The listing builds one solid part. Answer for the finished solid, in the listing's coordinates (mm). Face numbers are marked on the shaded views. A direction names the side the tool comes from. Give positions to 0.01 mm unless a question says otherwise; leave off trailing zeros. Order: outer loops, then holes, each group sorted by start corner. A loop starts at its lowest first (then second) coordinate and runs counter-clockwise, first axis right, second up.
Autodesk Inventor part; units mm, degrees
ref_plane "YZ Plane" through (0, 0, 0) normal (1, 0, 0) x (0, 1, 0)
ref_plane "XZ Plane" through (0, 0, 0) normal (0, 1, 0) x (-1, 0, 0)
ref_plane "XY Plane" through (0, 0, 0) normal (0, 0, 1) x (1, 0, 0)
sketch "Sketch1" plane through (0, 0, 0) normal (0, 1, 0) x (-1, 0, 0)
  line L0 (0, 0) -> (41.148, 0)
  line L1 (41.148, 0) -> (41.148, -20.32)
  line L2 (41.148, -20.32) -> (0, -20.32)
  line L3 (0, -20.32) -> (0, 0)
  circle A0 centre (45.212, -15.24) radius 2.0193
  circle A1 centre (-4.064, -15.24) radius 2.0193
  circle A2 centre (45.212, -5.08) radius 2.0193
  circle A3 centre (-4.064, -5.08) radius 2.0193
  line L4 (41.148, -9.652) -> (49.276, -9.652)
  line L5 (41.148, -10.668) -> (49.276, -10.668)
  line L6 (-13.1318, -9.652) -> (0, -9.652)
  line L7 (-13.1318, -10.668) -> (0, -10.668)
  line L8 (-13.1318, 3.81) -> (49.276, 3.81)
  line L9 (49.276, 3.81) -> (49.276, -24.13)
  line L10 (49.276, -24.13) -> (-13.1318, -24.13)
  line L11 (-13.1318, -30.9945) -> (-13.1318, 13.2145)
  line L12 (-6.155, -5.4575) -> (-6.0508, -5.4409)
  line L13 (-6.155, -5.4575) -> (-6.0508, -5.4409)
  line L14 (20.574, -20.32) -> (20.574, 0)
  circle A4 centre (10.668, -10.16) radius 6.604
  circle A5 centre (-6.7818, 6.8645) radius 2.0193
  circle A6 centre (30.6451, 9.4045) radius 2.0193
  circle A7 centre (30.6451, -27.1845) radius 2.0193
  line L15 (10.668, -30.9945) -> (34.4551, -30.9945)
  line L16 (-8.128, -30.9945) -> (34.4551, -30.9945)
  circle A8 centre (-9.3218, -27.1845) radius 2.0193
  line L17 (34.4424, -30.9945) -> (-13.1318, -30.9945)
  line L18 (34.4424, -24.13) -> (34.4424, -30.9945)
  line L19 (34.4424, 13.2145) -> (34.4424, 3.81)
  circle A9 centre (30.6451, 9.4045) radius 2.286
  circle A10 centre (-6.7818, 6.8645) radius 2.286
  circle A11 centre (-9.3218, -27.1845) radius 2.286
  circle A12 centre (30.6451, -27.1845) radius 2.286
  line L20 (34.4424, 3.81) -> (-13.1318, 3.81)
  line L21 (34.4424, 13.2145) -> (-13.1318, 13.2145)
  point P0 (20.574, -10.16)
  point P1 (34.4424, -30.9945)
  point P2 (-11.5492, -24.13)
  point P3 (-7.0944, -24.13)
  dimension "d0" = 41.148
  dimension "d1" = 20.32
  dimension "d4" = 4.0386
  dimension "d5" = 4.0386
  dimension "d18" = 4.064
  dimension "d19" = 4.064
  dimension "d52" = 8.128
  dimension "d53" = 13.1318
  dimension "d54" = 3.81
  dimension "d55" = 3.81
  dimension "d59" = 9.906
  dimension "d60" = 13.208
  dimension "d79" = 4.0386
  dimension "d80" = 4.0386
  dimension "d81" = 4.0386
  dimension "d82" = 4.0386
  dimension "d84" = 3.81
  dimension "d91" = 4.572
  dimension "d92" = 4.572
  dimension "d93" = 4.572
  dimension "d94" = 4.572
  dimension "d96" = 3.81
  dimension "d97" = 3.81
  dimension "d98" = 6.35
  dimension "d100" = 6.35
  dimension "d101" = 9.4045
  dimension "d102" = 47.5742
  dimension "d103" = 47.5742
extrude "Extrusion10" add sketch "Sketch1" along normal blind 11.811 contours L3 L6 L11 L8 L9 L4 L1 L0 | L0 L14 L2 L3 | L0 L1 L2 L14 | L3 L7 L11 L6 | L2 L1 L5 L9 L10 L11 L7 L3 | L4 L9 L5 L1 | L11 L21 L19 L8 | L10 L18 L15 L16 L17 L11
extrude "Extrusion11" cut sketch "Sketch1" along normal blind 10.16 contours L0 L14 L2 L3 | L0 L1 L2 L14
extrude "Extrusion12" cut sketch "Sketch1" along normal blind 2.032 contours L3 L7 L11 L6 | L4 L9 L5 L1
properties part number "Servo Mount"
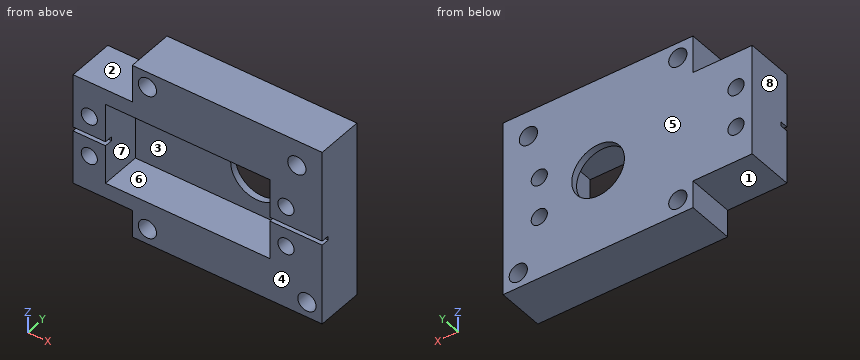
1) For a pull along X with two mould halves and no side action, classify the marked faces 5, 6, 7 and 8 as +X half, -X half, draft (parallel to the pull), parting line (faces both ways), or undercut.
Geometry says:
face 5: draft
face 6: undercut
face 7: undercut
face 8: -X half
2) Find section B-B (z = -5.08). Write down the section's boundary in (x, y).
Geometry says:
outline: (-49.28, 0) - (-47.23, 0) - (-47.23, 11.81) - (-49.28, 11.81) - close; (-43.19, 0) - (-41.15, 0) - (-41.15, 10.16) - (-14.89, 10.16) - (-14.89, 11.81) - (-43.19, 11.81) - close; (-6.45, 10.16) - (0, 10.16) - (0, 0) - (2.04, 0) - (2.04, 11.81) - (-6.45, 11.81) - close; (6.08, 0) - (13.13, 0) - (13.13, 11.81) - (6.08, 11.81) - close
3) Given P1, Ø3.5, axis at x = -38.5, y = 5, coming from the -Z side; P2, Ø3.5, axis at x = -30.65, z = -27.18, coming from the +Y side (3 decimals); P3, Ø3.5, axis at x = -41.5, y = 5, coming from the +Z side; P4, Ø2, axis at y = 5.5, z = 6, coming from the -X side, each flat-ended and moving along its own axis, determine where each tip first touches the part or whether it passes through.
Geometry says:
P1: stops at z = -24.13
P2: passes through
P3: stops at z = 3.81
P4: stops at x = -34.44
4) Find section A-A (y = 1). Count the separate pieces of the cut face and the enclosed holes in it, then the cut area to 3 significant figures.
Geometry says:
separate pieces: 2
enclosed holes: 8
area: 1,540 mm2
5) A tool of negligible diameter and unlimited length cuts with its end or side. For the marked faces 1, 2, 3 and 4, from which of +Z, -Z, +X, -X, +Y, -Y can it reach the whole face along a straight path? Write none if from no direction.
Geometry says:
face 1: -Z, -X, +Y, -Y
face 2: +Z, -X, +Y, -Y
face 3: -Y
face 4: +Z, -Z, +X, -X, -Y
6) Find section D-D (x = -31). Write down the section's boundary in (y, z).
Geometry says:
outline: (0, -30.99) - (11.81, -30.99) - (11.81, -29.44) - (0, -29.44) - close; (0, -24.93) - (11.81, -24.93) - (11.81, 7.15) - (0, 7.15) - (0, 0) - (10.16, 0) - (10.16, -20.32) - (0, -20.32) - close; (0, 11.66) - (11.81, 11.66) - (11.81, 13.21) - (0, 13.21) - close
7) Straight lines are drawn through the part: probe 1 along X at (y, z) = (2.25, -3); probe 2 along Z at (x, y) = (-13.5, 2.5); probe 3 along X at (y, z) = (10, -17). For each, find the intervals that lie inside material, in ascending order.
Geometry says:
probe 1: x = -49.28 to -41.15, 0 to 13.13
probe 2: z = -30.99 to -20.32, 0 to 13.21
probe 3: x = -49.28 to -46.2, -44.22 to -41.15, 0 to 3.07, 5.05 to 13.13
